from build123d import *

# Parameters (mm, degrees)
F1_DEPTH = 25.4


with BuildPart() as f1:
    # F0 (on Front) → F1 (new body)
    with BuildSketch(Plane.XZ):
        with BuildLine():
            Line((-1.7960512242, 1.7960512242), (-24.3212742751, 24.3212742751))
            ThreePointArc((-24.3212742751, 24.3212742751), (-25.1022111456, 23.1678047767), (-25.3989050096, 21.8068025612))
            Line((-25.3989050096, 21.8068025612), (-3.5921024484, 0))
            Line((-3.5921024484, 0), (-1.7960512242, 1.7960512242))
        make_face()
        with BuildLine():
            Line((0, 3.5921024484), (-21.8068025612, 25.3989050096))
            ThreePointArc((-21.8068025612, 25.3989050096), (-23.1678047767, 25.1022111456), (-24.3212742751, 24.3212742751))
            Line((-24.3212742751, 24.3212742751), (-1.7960512242, 1.7960512242))
            Line((-1.7960512242, 1.7960512242), (0, 3.5921024484))
        make_face()
        Polygon((0, 0), (-1.7960512242, 1.7960512242), (-3.5921024484, 0), (-1.7960512242, -1.7960512242), align=None)
        Polygon((1.7960512242, 1.7960512242), (0, 3.5921024484), (-1.7960512242, 1.7960512242), (0, 0), align=None)
        Polygon((3.5921024484, 0), (1.7960512242, 1.7960512242), (0, 0), (1.7960512242, -1.7960512242), align=None)
        Polygon((1.7960512242, -1.7960512242), (0, 0), (-1.7960512242, -1.7960512242), (0, -3.5921024484), align=None)
        with BuildLine():
            ThreePointArc((24.3212742751, 24.3212742751), (23.1678047767, 25.1022111456), (21.8068025612, 25.3989050096))
            Line((21.8068025612, 25.3989050096), (0, 3.5921024484))
            Line((0, 3.5921024484), (1.7960512242, 1.7960512242))
            Line((1.7960512242, 1.7960512242), (24.3212742751, 24.3212742751))
        make_face()
        with BuildLine():
            ThreePointArc((25.3989050096, 21.8068025612), (25.1022111456, 23.1678047767), (24.3212742751, 24.3212742751))
            Line((24.3212742751, 24.3212742751), (1.7960512242, 1.7960512242))
            Line((1.7960512242, 1.7960512242), (3.5921024484, 0))
            Line((3.5921024484, 0), (25.3989050096, 21.8068025612))
        make_face()
        with BuildLine():
            Line((25.3989050096, -21.8068025612), (3.5921024484, 0))
            Line((3.5921024484, 0), (1.7960512242, -1.7960512242))
            Line((1.7960512242, -1.7960512242), (24.3212742751, -24.3212742751))
            ThreePointArc((24.3212742751, -24.3212742751), (25.1022111456, -23.1678047767), (25.3989050096, -21.8068025612))
        make_face()
        with BuildLine():
            Line((-1.7960512242, -1.7960512242), (-3.5921024484, 0))
            Line((-3.5921024484, 0), (-25.3989050096, -21.8068025612))
            ThreePointArc((-25.3989050096, -21.8068025612), (-25.1022111456, -23.1678047767), (-24.3212742751, -24.3212742751))
            Line((-24.3212742751, -24.3212742751), (-1.7960512242, -1.7960512242))
        make_face()
        with BuildLine():
            Line((0, -3.5921024484), (-1.7960512242, -1.7960512242))
            Line((-1.7960512242, -1.7960512242), (-24.3212742751, -24.3212742751))
            ThreePointArc((-24.3212742751, -24.3212742751), (-23.1678047767, -25.1022111456), (-21.8068025612, -25.3989050096))
            Line((-21.8068025612, -25.3989050096), (0, -3.5921024484))
        make_face()
        with BuildLine():
            Line((24.3212742751, -24.3212742751), (1.7960512242, -1.7960512242))
            Line((1.7960512242, -1.7960512242), (0, -3.5921024484))
            Line((0, -3.5921024484), (21.8068025612, -25.3989050096))
            ThreePointArc((21.8068025612, -25.3989050096), (23.1678047767, -25.1022111456), (24.3212742751, -24.3212742751))
        make_face()
    extrude(amount=F1_DEPTH)


solid = f1.part
Model file for the job. Use its own axes, mm. A direction names the side the tool comes from. Round coordinates to 2 decimals unless told otherwise and drop trailing zeros. Order: outer loops, then holes, each group sorted by start corner. A loop starts at its lowest first (then second) coordinate and runs counter-clockwise, first axis right, second up.
(1) Band-saw the part on D-D (x = -2). List the corners of the cut face in (y, z), then the cut area to 3 significant figures.
(2) Band-saw the part on C-C (x = -7.5). List the corners of the cut face in (y, z).
(3) 3-axis set-ups, long thin cutter, end or side, ignore diameter. For faces 1 (the face through (-14.65, -12.52, 11.06)), 2 (the face through (-10.75, -12.52, 14.34)), 3 (the face through (14.65, -12.52, -11.06)), 4 (the face through (-11.06, -12.52, -14.65)), 5 (the face through (0, -25.4, 0)): which of +Z, -Z, +X, -X, +Y, -Y reach the whole face in a straight line?
(4) Pull direction Z, two halves, no side cores. Call faces 6 (the face through (-14.34, -12.52, -10.75)), 7 (the face through (0, 0, 0)), 8 (the face through (10.75, -12.52, -14.34)), 9 (the face through (14.34, -12.52, 10.75)): released by +Z, released by -Z, zero draft, split by the parting line, or undercut.
(5) Drill centre lines: line 1 (Z direction, x = 7.5, y = -22); line 2 (X direction, y = -15.75, z = 11); line 3 (Z direction, x = 4, y = -20). Where is each one in solid material? Low to high.
(6) Pin check, flat tips, straight feed: pin 1 (1 mm diameter, centred on y = -19, z = 11.5, fed in from -X); pin 2 (1 mm diameter, centred on y = -5, z = -16, fed in from +X); pin 3 (10 mm diameter, centred on x = -4.5, y = -8.5, fed in from +Z). Stop position of each tip, or through.
(7) Band-saw the part on A-A (y = -18). List the corners of the cut face in (x, z), then the cut area to 3 significant figures.
(8) Band-saw the part on B-B (z = 6). List the corners of the cut face in (x, y).
Verdict:
1. outline: (-25.4, -5.59) - (0, -5.59) - (0, 5.59) - (-25.4, 5.59) - close
1. area: 284 mm2
2. outline: (-25.4, -11.09) - (0, -11.09) - (0, -3.91) - (-25.4, -3.91) - close; (-25.4, 3.91) - (0, 3.91) - (0, 11.09) - (-25.4, 11.09) - close
3. face 1: -X, +Y, -Y
3. face 2: +Z, +Y, -Y
3. face 3: +X, +Y, -Y
3. face 4: -Z, +Y, -Y
3. face 5: +Z, -Z, +X, -X, -Y
4. face 6: undercut
4. face 7: zero draft
4. face 8: released by -Z
4. face 9: undercut
5. line 1: z = -11.09 to -3.91, 3.91 to 11.09
5. line 2: x = -14.59 to -7.41, 7.41 to 14.59
5. line 3: z = -7.59 to -0.41, 0.41 to 7.59
6. pin 1: stops at x = -15.59
6. pin 2: stops at x = 20.09
6. pin 3: stops at z = 13.09
7. outline: (-25.4, -21.81) arc R3.68 ccw to (-21.81, -25.4) - (0, -3.59) - (21.81, -25.4) arc R3.68 ccw to (25.4, -21.81) - (3.59, 0) - (25.4, 21.81) arc R3.68 ccw to (21.81, 25.4) - (0, 3.59) - (-21.81, 25.4) arc R3.68 ccw to (-25.4, 21.81) - (-3.59, 0) - close
7. area: 667 mm2
8. outline: (-9.59, -25.4) - (-2.41, -25.4) - (-2.41, 0) - (-9.59, 0) - close; (2.41, -25.4) - (9.59, -25.4) - (9.59, 0) - (2.41, 0) - close
